Build history of the part. All positions in model axes, mm. A direction names the side the tool comes from. Coordinates: 2 decimals unless noted, no trailing zeros. Loops run counter-clockwise (first coordinate to the right, second up) from the corner with the lowest first, then second, coordinate; pieces in that order, holes last. Notation, with made-up numbers: (29, 47) - (76, 47) arc R23 ccw to (76, 79) - close; hole circle Ø5 at (-26, 59). An arc over 180 degrees is marked (long way). One line per item, written item: value.
```python
from build123d import *

# Parameters (mm, degrees)
BOSS_EXTRUDE1_DEPTH = 50
SKETCH2_W           = 37
SKETCH2_H           = 33.3
BOSS_EXTRUDE2_DEPTH = 3
SKETCH3_W           = 20
SKETCH3_H           = 7
CUT_EXTRUDE1_DEPTH  = 50


with BuildPart() as part:
    # Sketch1 → Boss-Extrude1 (new body, symmetric)
    with BuildSketch(Plane(origin=(0, 0, 0), x_dir=(0, 0, -1), z_dir=(1, 0, 0))):
        Polygon((16, 0), (18, 0), (18, -33.3), (-19, -33.3), (-19, 0), (-17, 0), (-17, -31.3), (16, -31.3), align=None)
    extrude(amount=BOSS_EXTRUDE1_DEPTH, both=True)

    # Sketch2 → Boss-Extrude2 (add)
    with BuildSketch(Plane.ZY.offset(50)):
        with Locations((0.5, -16.65)):
            Rectangle(SKETCH2_W, SKETCH2_H)
    extrude(amount=-BOSS_EXTRUDE2_DEPTH)

    # Sketch3 → Cut-Extrude1 (cut)
    with BuildSketch(Plane(origin=(0, 0, 0), x_dir=(1, 0, 0), z_dir=(0, 1, 0))):
        with Locations((-30, -13.5)):
            Rectangle(SKETCH3_W, SKETCH3_H)
        with Locations((5, -13.5)):
            Rectangle(SKETCH3_W, SKETCH3_H)
        with Locations((-30, 12.5)):
            Rectangle(SKETCH3_W, SKETCH3_H)
        with Locations((5, 12.5)):
            Rectangle(SKETCH3_W, SKETCH3_H)
    extrude(amount=-CUT_EXTRUDE1_DEPTH, mode=Mode.SUBTRACT)


solid = part.part
```
Item 1: Tool access for faces 1 (the face through (1, -17, 19)), 2 (the face through (2, -31.3, 1)), 3 (the face through (15, -32, -12)): list every direction of +Z, -Z, +X, -X, +Y, -Y with a clear straight run to the whole face (end or side of a thin tool).
Check result:
face 1: +Z, +X, -X, +Y, -Y
face 2: +X, +Y
face 3: +Y, -Y
Item 2: Cut at B-B, the plane z = 15.5. Write the cut outline in (x, y).
Check result:
outline: (-50, -33.3) - (-40, -33.3) - (-40, -31.3) - (-47, -31.3) - (-47, 0) - (-50, 0) - close; (-20, -33.3) - (-5, -33.3) - (-5, -31.3) - (-20, -31.3) - close; (15, -33.3) - (50, -33.3) - (50, -31.3) - (15, -31.3) - close
Item 3: Pull direction X, two halves, no side cores. Call faces 4 (the face through (-50, -16, 0)), 5 (the face through (1, -16, -18)), 6 (the face through (-20, -32, 14)), 7 (the face through (-40, -32, -12)): released by +X, released by -X, zero draft, split by the parting line, or undercut.
Check result:
face 4: released by -X
face 5: zero draft
face 6: undercut
face 7: undercut
Item 4: Probe probe 1 along Z at (x, y) = (-2.5, -25.5); probe 2 along Y at (x, z) = (44.5, -7); probe 3 along X at (y, z) = (-14, -12). List the from-to ranges inside material, lowest first. Write a range as from..to.
Check result:
probe 1: z = -18..-16, 17..19
probe 2: y = -33.3..-31.3
probe 3: x = -50..-47
Item 5: Drop flat-ended pins along their axis: P1, Ø16.5, axis at x = -4, z = -0.5, coming from the +Y side; P2, Ø6, axis at y = -19, z = 5, coming from the +X side. Give the stop position or say it passes through.
Check result:
P1: stops at y = -31.3
P2: stops at x = -47
Item 6: Cut at C-C, the plane y = -7.5. Write the cut outline in (x, z).
Check result:
outline: (-50, -18) - (50, -18) - (50, -16) - (-47, -16) - (-47, 17) - (50, 17) - (50, 19) - (-50, 19) - close
Item 7: Cut at A-A, the plane x = -34. Write the cut outline in (y, z).
Check result:
outline: (-33.3, -18) - (0, -18) - (0, -16) - (-33.3, -16) - close; (-33.3, -9) - (-31.3, -9) - (-31.3, 10) - (-33.3, 10) - close; (-33.3, 17) - (0, 17) - (0, 19) - (-33.3, 19) - close
Item 8: Cut at D-D, the plane x = 22. Write the cut outline in (y, z).
Check result:
outline: (-33.3, -18) - (0, -18) - (0, -16) - (-31.3, -16) - (-31.3, 17) - (0, 17) - (0, 19) - (-33.3, 19) - close
